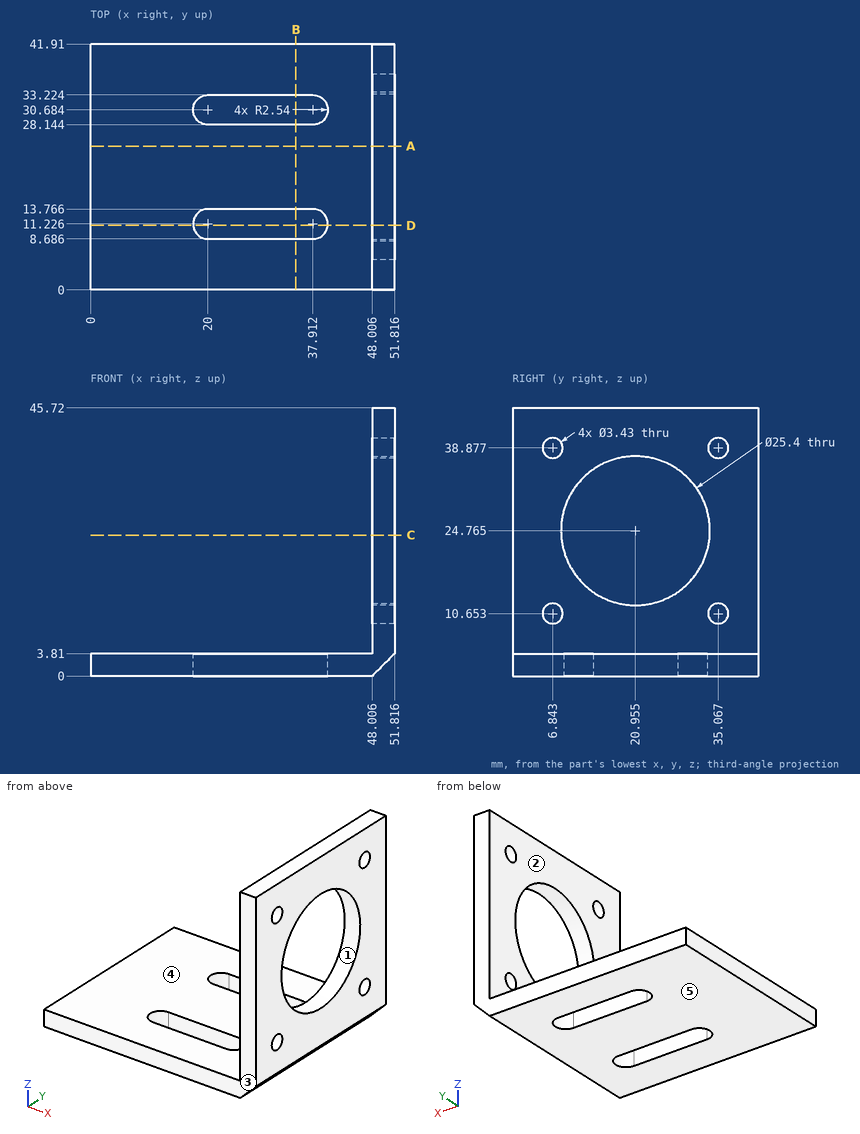
For this review, use the dimensioned drawing (mm, ordinates from the lowest corner) and the shaded views. A direction names the side the tool comes from. Round coordinates to 2 decimals unless told otherwise and drop trailing zeros. Loops run counter-clockwise (first coordinate to the right, second up) from the corner with the lowest first, then second, coordinate; pieces in that order, holes last. Notation, with made-up numbers: M 5,46.25 L 48,46.25 A31 ccw 48,73.25 Z; hole C 6.25,15.25 d10. An arc over 180 degrees is marked long. Answer as CSV lines item,"result".
1. Insertion check: pin 1 Ø4 at (y, z) = (6.84, 10.65) entering from -X; pin 2 Ø20.5 at (y, z) = (20.955, 24.765) entering from +X; pin 3 Ø3 at (x, y) = (40, 19) entering from +Z. Each pin has a flat end and moves straight along its axis. Give the tip position at first contact, or say it passes through.
Outcome:
pin 1,"stops at x = 48.01"
pin 2,"passes through"
pin 3,"stops at z = 3.81"
2. We need section B-B (x = 35). Give the boundary of the cut face in (y, z).
Outcome:
outline,"M 0,0 L 8.69,0 L 8.69,3.81 L 0,3.81 Z; M 13.77,0 L 28.14,0 L 28.14,3.81 L 13.77,3.81 Z; M 33.22,0 L 41.91,0 L 41.91,3.81 L 33.22,3.81 Z"
3. For the marked faces 4 and 5, list the 3-axis set-ups (+Z, -Z, +X, -X, +Y, -Y) from which the entire face can be reached by the end or side of a thin tool; tool diameter is ignored.
Outcome:
face 4,"+Z, -X, +Y, -Y"
face 5,"-Z, +X, -X, +Y, -Y"
4. Draft analysis for pull direction Y (two halves, no side actions). For the marked faces 1, 2 and 3, state which applies: pulls with the +Y half, pulls with the -Y half, needs draft (parallel to the pull), parting line crosses it, or undercut.
Outcome:
face 1,"undercut"
face 2,"needs draft"
face 3,"pulls with the -Y half"
5. To check wall thickness, follow L1, parallel to Z at x = 24.5, y = 26; L2, parallel to Y at x = 49.5, z = 22; L3, parallel to X at y = 38, z = 14. State the ranges of each line that lie inside material, in increasing order. Write a range as [from, to].
Outcome:
L1,"z = [0, 3.81]"
L2,"y = [0, 8.56], [33.35, 41.91]"
L3,"x = [48.01, 51.82]"
6. We need section C-C (z = 24). Give the boundary of the cut face in (x, y), plus the area to 3 significant figures.
Outcome:
outline,"M 48.01,0 L 51.82,0 L 51.82,8.28 L 48.01,8.28 Z; M 48.01,33.63 L 51.82,33.63 L 51.82,41.91 L 48.01,41.91 Z"
area,"63.1 mm2"
7. We need section A-A (y = 24.5). Give the boundary of the cut face in (x, z).
Outcome:
outline,"M 0,0 L 48.01,0 L 51.82,3.81 L 51.82,12.57 L 48.01,12.57 L 48.01,3.81 L 0,3.81 Z; M 48.01,36.96 L 51.82,36.96 L 51.82,45.72 L 48.01,45.72 Z"
8. We need section D-D (y = 11). Give the boundary of the cut face in (x, z).
Outcome:
outline,"M 0,0 L 17.47,0 L 17.47,3.81 L 0,3.81 Z; M 40.44,0 L 48.01,0 L 51.82,3.81 L 51.82,16.88 L 48.01,16.88 L 48.01,3.81 L 40.44,3.81 Z; M 48.01,32.65 L 51.82,32.65 L 51.82,45.72 L 48.01,45.72 Z"
